The figure shows three views and two pictorial views of one solid part (mm, origin at its lowest corner). Answer the questions. Round coordinates to 2 decimals unless told otherwise and drop trailing zeros. Order: outer loops, then holes, each group sorted by start corner. A loop starts at its lowest first (then second) coordinate and runs counter-clockwise, first axis right, second up. Notation, with made-up numbers: (-3.5, 61.25) -> (44.5, 61.25) arc R25 cw to (44.5, 88.25) -> close; hole circle Ø10 at (40, 37.5). An arc over 180 degrees is marked (long way). Return JSON: item names as keys, results as strings. Group by question number.
(1) The part is cut by section C-C (z = 2.1). Count the separate pieces of the cut face and the enclosed holes in it, plus the area to 3 significant figures.
(2) The part is cut by section D-D (x = 5). Determine the outline of the cut face in (y, z), plus the area to 3 significant figures.
(3) The part is cut by section A-A (y = 12). Determine the outline of the cut face in (x, z), plus the area to 4 significant figures.
(4) Consider line 1 (Y direction, x = 64, z = 2.4); line 2 (X direction, y = 15, z = 4.35); line 3 (Y direction, x = 61, z = 2.25). Determine where each line is inside the solid, lowest interval first. Write a range as [from, to].
(5) The part is cut by section B-B (x = 39). Determine the outline of the cut face in (y, z), plus the area to 3 significant figures.
(6) Determine the mould class of the marked faces 1, 2 and 3 for opening direction Y: +Y half, -Y half, draft (parallel to the pull), parting line (faces both ways), or undercut.
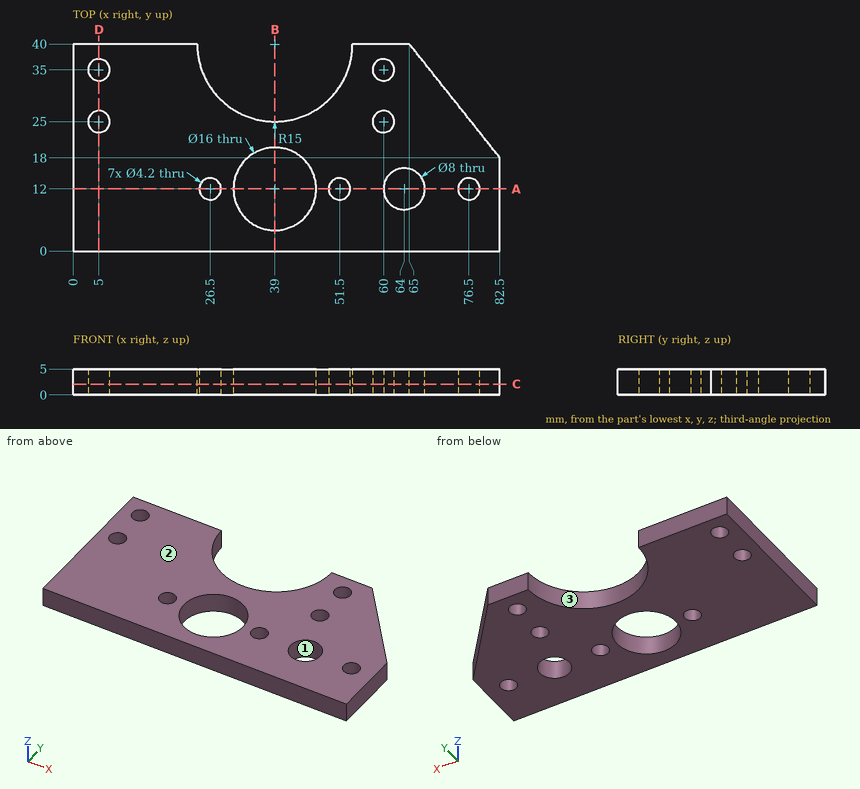
Answer below:
{
 "1": {"separate pieces": "1", "enclosed holes": "9", "area": "2,410 mm²"},
 "2": {"outline": "(0, 0) -> (22.9, 0) -> (22.9, 5) -> (0, 5) -> close; (27.1, 0) -> (32.9, 0) -> (32.9, 5) -> (27.1, 5) -> close; (37.1, 0) -> (40, 0) -> (40, 5) -> (37.1, 5) -> close", "area": "158 mm²"},
 "3": {"outline": "(0, 0) -> (24.4, 0) -> (24.4, 5) -> (0, 5) -> close; (28.6, 0) -> (31, 0) -> (31, 5) -> (28.6, 5) -> close; (47, 0) -> (49.4, 0) -> (49.4, 5) -> (47, 5) -> close; (53.6, 0) -> (60, 0) -> (60, 5) -> (53.6, 5) -> close; (68, 0) -> (74.4, 0) -> (74.4, 5) -> (68, 5) -> close; (78.6, 0) -> (82.5, 0) -> (82.5, 5) -> (78.6, 5) -> close", "area": "229.5 mm²"},
 "4": {"line 1": "y = [0, 8], [16, 40]", "line 2": "x = [0, 31.58], [46.42, 61.35], [66.65, 82.5]", "line 3": "y = [0, 9.35], [14.65, 23.15], [26.85, 33.15], [36.85, 40]"},
 "5": {"outline": "(0, 0) -> (4, 0) -> (4, 5) -> (0, 5) -> close; (20, 0) -> (25, 0) -> (25, 5) -> (20, 5) -> close", "area": "45.0 mm²"},
 "6": {"face 1": "undercut", "face 2": "draft", "face 3": "+Y half"}
}
